Answer from the drawing. Dimensions are ordinates in mm from the lowest x, y and z of the part. A direction names the side the tool comes from. Give positions to 0.01 mm unless a question says otherwise; leave off trailing zeros. Loops run counter-clockwise (first coordinate to the right, second up) from the corner with the lowest first, then second, coordinate; pieces in that order, holes last.
Item 1: A tool of negligible diameter and unlimited length cuts with its end or side. For the marked faces 1, 2 and 3, from which of +Z, -Z, +X, -X, +Y, -Y can it reach the whole face along a straight path? Write none if from no direction.
Item 2: Section A-A, the plane z = 3.75 is taken. Give the vertices of the cut face in (x, y).
Item 3: Section D-D, the plane z = 7 is taken. Give the vertices of the cut face in (x, y).
Item 4: Consider line 1 along Y through (x, z) = (20, 4.75); line 2 along Z through (x, y) = (15.5, 23); line 3 along Y through (x, z) = (20, 2.5) (1 decimal). Determine where each line is inside the solid, lowest interval first.
Item 5: Each of these flat-tipped pins is pushed along its axis until it touches: pin 1 Ø4 at (x, y) = (12.5, 12) entering from +Z; pin 2 Ø1.5 at (x, z) = (27, 6.5) entering from -Y; pin 3 Ø5 at (x, z) = (10.5, 7) entering from -Y. Where does it stop, or does it pass through?
Item 6: Section C-C, the plane x = 7 is taken. Give the vertices of the cut face in (y, z).
Item 7: Section B-B, the plane y = 28.5 is taken. Give the vertices of the cut face in (x, z).
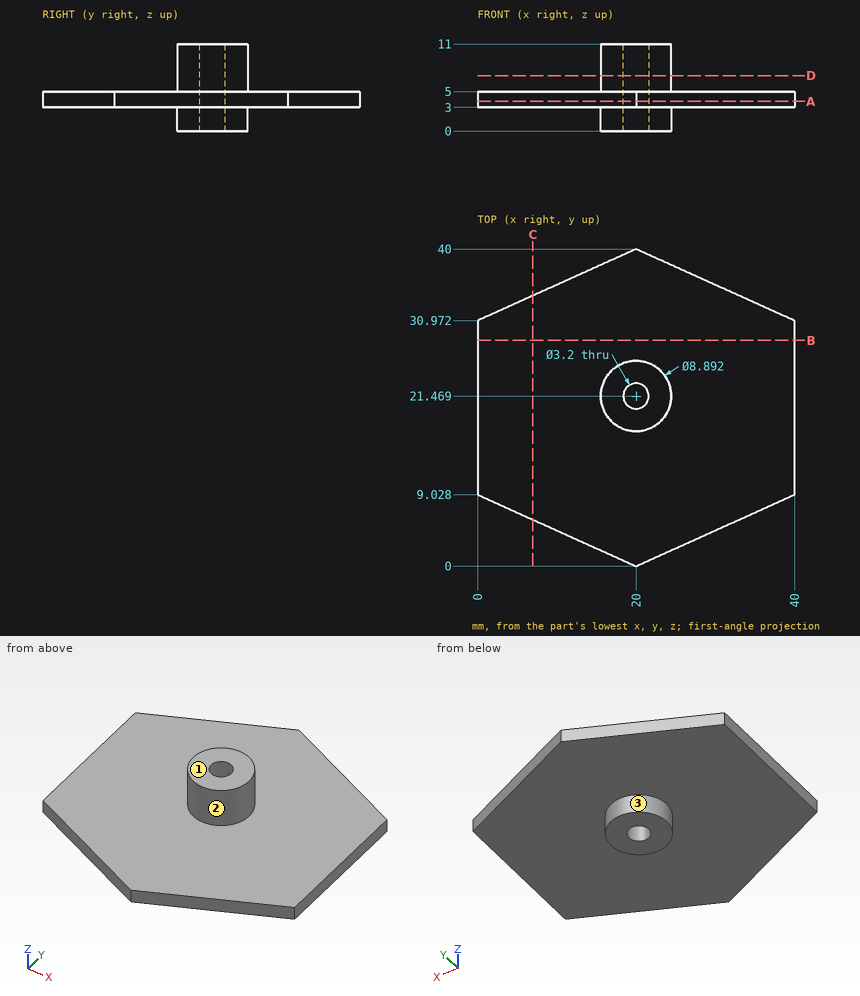
Worked answers:
1. face 1: +Z, +X, -X, +Y, -Y
1. face 2: +Z
1. face 3: -Z
2. outline: (0, 9.03) - (20, 0) - (40, 9.03) - (40, 30.97) - (20, 40) - (0, 30.97) - close; hole circle Ø3.2 at (20, 21.47)
3. outline: circle Ø8.89 at (20, 21.47); hole circle Ø3.2 at (20, 21.47)
4. line 1: y = 0 to 19.87, 23.07 to 40
4. line 2: z = 3 to 5
4. line 3: y = 17 to 19.9, 23.1 to 25.9
5. pin 1: stops at z = 5
5. pin 2: passes through
5. pin 3: stops at y = 3.61
6. outline: (5.87, 3) - (34.13, 3) - (34.13, 5) - (5.87, 5) - close
7. outline: (0, 3) - (40, 3) - (40, 5) - (0, 5) - close
